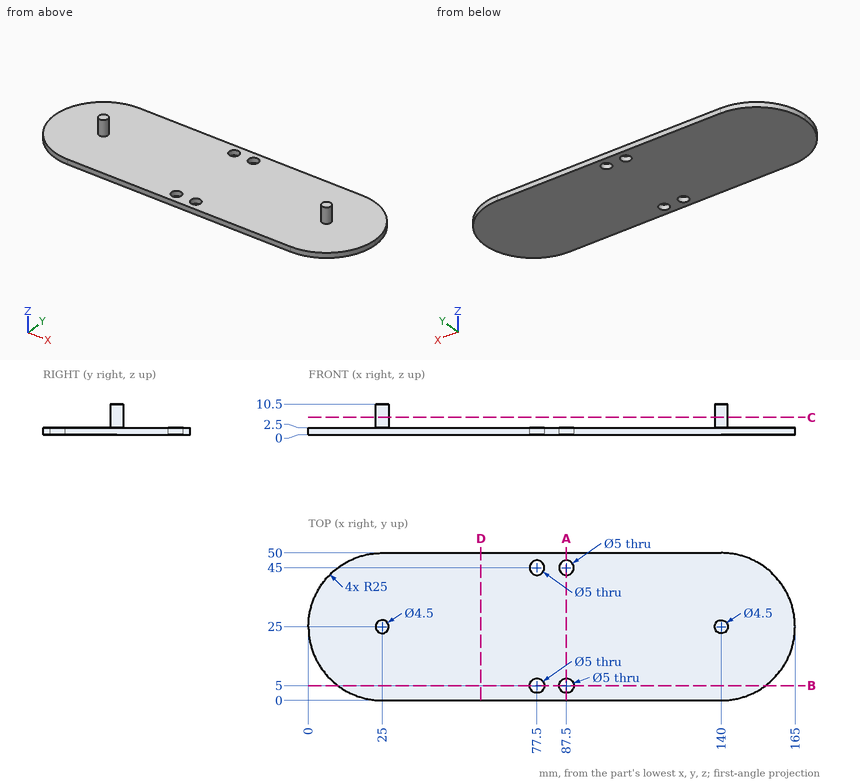
Part print with two shaded views. Sizes in mm from the minimum x, y, z corner. Give positions to 0.01 mm unless a question says otherwise; leave off trailing zeros. Order: outer loops, then holes, each group sorted by start corner. A loop starts at its lowest first (then second) coordinate and runs counter-clockwise, first axis right, second up. Notation, with made-up numbers: (73.25, 58.5) - (116.25, 58.5) arc R10 ccw to (116.25, 66.5) - close; hole circle Ø3 at (22.25, 10). An arc over 180 degrees is marked (long way). Write each question's results on one line, items separated by ' | '.
1. Saw through at B-B on y = 5. List the corners of the cut face in (x, z).
Calculated:
outline: (10, 0) - (75, 0) - (75, 2.5) - (10, 2.5) - close; (80, 0) - (85, 0) - (85, 2.5) - (80, 2.5) - close; (90, 0) - (155, 0) - (155, 2.5) - (90, 2.5) - close
2. Pin check, flat tips, straight feed: pin 1 (8 mm diameter, centred on x = 61, y = 14.5, fed in from +Z); pin 2 (4 mm diameter, centred on x = 77.5, y = 5, fed in from -Z); pin 3 (6 mm diameter, centred on y = 34.5, z = 1.5, fed in from +X); pin 4 (6 mm diameter, centred on y = 10, z = 2, fed in from +X). Stop position of each tip, or through.
Calculated:
pin 1: stops at z = 2.5 | pin 2: passes through | pin 3: stops at x = 164.14 | pin 4: stops at x = 161.93
3. Saw through at A-A on x = 87.5. List the corners of the cut face in (y, z), and give its area (3 significant figures).
Calculated:
outline: (0, 0) - (2.5, 0) - (2.5, 2.5) - (0, 2.5) - close; (7.5, 0) - (42.5, 0) - (42.5, 2.5) - (7.5, 2.5) - close; (47.5, 0) - (50, 0) - (50, 2.5) - (47.5, 2.5) - close | area: 100 mm2
4. Probe L1, parallel to Y at x = 87.5, z = 0.7; L2, parallel to Z at x = 22, y = 45; L3, parallel to X at y = 34, z = 2.25. List the from-to ranges inside material, lowest first. Write a range as from..to.
Calculated:
L1: y = 0..2.5, 7.5..42.5, 47.5..50 | L2: z = 0..2.5 | L3: x = 1.68..163.32
5. Saw through at C-C on z = 6. List the corners of the cut face in (x, y), and give its area (3 significant figures).
Calculated:
outline: circle Ø4.5 at (25, 25); circle Ø4.5 at (140, 25) | area: 31.8 mm2
6. Saw through at D-D on x = 58.5. List the corners of the cut face in (y, z), and give its area (3 significant figures).
Calculated:
outline: (0, 0) - (50, 0) - (50, 2.5) - (0, 2.5) - close | area: 125 mm2
